Autodesk Inventor part; units mm, degrees
ref_plane "YZ Plane" through (0, 0, 0) normal (1, 0, 0) x (0, 1, 0)
ref_plane "XZ Plane" through (0, 0, 0) normal (0, 1, 0) x (-1, 0, 0)
ref_plane "XY Plane" through (0, 0, 0) normal (0, 0, 1) x (1, 0, 0)
sketch "Náčrt1" plane through (0, 0, 0) normal (0, 1, 0) x (-1, 0, 0)
  line L0 (20, -5) -> (0, -5)
  line L1 (20, -5) -> (20, -11)
  line L2 (20, -11) -> (6, -16.3741)
  line L3 (6, -16.3741) -> (6, -35.9212)
  line L4 (0, 0) -> (-43.8955, 0)
  arc A0 (20, -55) -> (6, -35.9212) centre (0, -55) ccw
  line L5 (0, 0) -> (0, -73.1539)
  line L6 (20, -55) -> (15, -55)
  arc A1 (15, -55) -> (0, -40) centre (0, -55) ccw
  line L7 (24.648, -55) -> (-37.389, -55)
  line L8 (20, -55) -> (20, -66.6969)
  line L9 (-20, -5) -> (0, -5)
  line L10 (-20, -5) -> (-20, -11)
  line L11 (-20, -11) -> (-6, -16.3741)
  line L12 (-6, -16.3741) -> (-6, -35.9212)
  arc A2 (-6, -35.9212) -> (-20, -55) centre (0, -55) ccw
  line L13 (-20, -55) -> (-15, -55)
  arc A3 (0, -40) -> (-15, -55) centre (0, -55) ccw
  point P0 (0, -53)
  dimension "d1" = 111
  dimension "d3" = 10
  dimension "d63" = 20
  dimension "d64" = 15
  dimension "d65" = 12
  dimension "d67" = 80
  dimension "d68" = 6
revolve "Rotace1" add sketch "Náčrt1" angle 360 about axis through (0, 0, 0) along (1, 0, 0) contours L1 L2 L3 A0 L6 A1 L5 L0 | L5 A3 L7 A2 L12 L11 L10 L9
properties part number "pulley_dc"
CAD build for the part. Positions are in the model's coordinates, mm. A direction names the side the tool comes from. Coordinates: 2 decimals unless noted, no trailing zeros. Write each loop counter-clockwise with the first axis right and the second up, starting at its lowest first coordinate (ties: lowest second). Pieces come first, ordered by that corner, then holes. Notation, with made-up numbers: M -32.75,-28 L -20.75,-28 A7 cw -20.75,-24 Z; hole C 3.25,62.25 d7. An arc over 180 degrees is marked long. Answer as a JSON object with one key per item and string values. Group by question number.
1) Pin check, flat tips, straight feed: pin 1 Ø1.5 at (y, z) = (-25, -11.5) entering from -X; pin 2 Ø4 at (x, z) = (-7.5, -33.5) entering from -Y; pin 3 Ø1 at (x, z) = (2, 7.5) entering from -Y; pin 4 Ø9 at (y, z) = (0, 0) entering from -X. Stop position of each tip, or through.
2) Wall check: line 1 (Y direction, x = 9, z = -4); line 2 (Y direction, x = 10.5, z = 0.5); line 3 (X direction, y = 12, z = -18.5). Give the ranges that are in metal, low to high. Write a range as from..to.
3) Tool access for faces 4 (the face through (-20, -5, -2)), 5 (the face through (-6, -7, -15)), 6 (the face through (6, -7, -15)): list every direction of +Z, -Z, +X, -X, +Y, -Y with a clear straight run to the whole face (end or side of a thin tool).
4) Saw through at A-A (y = 0). Write the cut outline in (x, z), plus the area to 3 significant figures.
5) Saw through at C-C (x = 17). Write the cut outline in (y, z), plus the area to 3 significant figures.
6) Saw through at D-D (x = -2). Write the cut outline in (y, z).
7) Mould opens along Y. For faces 1 (the face through (17.535, -53.692, 11.923)), 2 (the face through (20, -5, -2)), 3 (the face through (-0.28, 4.88, 1.08)) say: +Y half, -Y half, draft (parallel to the pull), parting line (faces both ways), or undercut.
Values follow:
{
 "1": {"pin 1": "stops at x = -6", "pin 2": "stops at y = -28.53", "pin 3": "stops at y = -39.55", "pin 4": "passes through"},
 "2": {"line 1": "y = -42.81..-36.92, -14.69..-3, 3..14.69, 36.92..42.81", "line 2": "y = -44.29..-37.97, -14.64..-4.97, 4.97..14.64, 37.97..44.29", "line 3": "x = -6..6"},
 "3": {"face 4": "+Z, -Z, -X, +Y, -Y", "face 5": "-X", "face 6": "+X"},
 "4": {"outline": "M -20,-55 L -15,-55 A15 cw 15,-55 L 20,-55 A20 ccw 6,-35.92 L 6,-16.37 L 20,-11 L 20,-5 L -20,-5 L -20,-11 L -6,-16.37 L -6,-35.92 A20 ccw Z; M -20,5 L 20,5 L 20,11 L 6,16.37 L 6,35.92 A20 ccw 20,55 L 15,55 A15 cw -15,55 L -20,55 A20 ccw -6,35.92 L -6,16.37 L -20,11 Z", "area": "1,760 mm2"},
 "5": {"outline": "C 0,0 d110; C 0,0 d24.3; hole C 0,0 d88.93; hole C 0,0 d10", "area": "3,680 mm2"},
 "6": {"outline": "C 0,0 d80.27; hole C 0,0 d10"},
 "7": {"face 1": "parting line", "face 2": "draft", "face 3": "undercut"}
}
